Design review of the part built by this model. Coordinates are the model's own, in mm. A direction names the side the tool comes from. Coordinates: 2 decimals unless noted, no trailing zeros. Write each loop counter-clockwise with the first axis right and the second up, starting at its lowest first coordinate (ties: lowest second). Pieces come first, ordered by that corner, then holes. Notation, with made-up numbers: (48, -8) -> (72, -8) arc R17 cw to (72, 17) -> close; hole circle Ø5 at (5, 59.5). An arc over 180 degrees is marked (long way). One line per question, with ' | ' between items. Start each with the question number.
Q1. Add section A-A on x = -1.7. State the section outline as (y, z) points.
Q2. Add section C-C on y = 6.5. State the section outline as (x, z) points.
Q3. Add section B-B on z = 30. State the section outline as (x, y) points, and give its area (3 significant figures).
Q4. Add section D-D on y = 33. State the section outline as (x, z) points.
Q5. For faces 4 (the cylindrical face through (-1.014, 27.683, -34.52)), 5 (the cylindrical face through (-1.014, 37.683, 53.485)), list the 3-axis set-ups (+Z, -Z, +X, -X, +Y, -Y) from which the entire face can be reached by the end or side of a thin tool; tool diameter is ignored.
Q6. Draft analysis for pull direction Y (two halves, no side actions). For faces 1 (the flat face through (-1, 39.325, -1)), 2 (the cylindrical face through (-1.014, -11.689, 9.026)), 3 (the flat face through (-2, 30, 1)), state which applies: pulls with the +Y half, pulls with the -Y half, needs draft (parallel to the pull), parting line crosses it, or undercut.
Q7. Wall thickness on probe 1 along Y at (x, z) = (-0.6, 1.5); probe 2 along Z at (x, y) = (-1.15, 17); probe 3 along Y at (x, z) = (-1.2, 10.5): over which ranges is each line inside the solid? List them lowest first.
from build123d import *

# Parameters (mm, degrees)
BASE_FLANGE1_DEPTH = 2
FILLET1_R          = 3


# Sheet-metal steps are written as plain solids
with BuildPart() as part:
    # Sketch1 → Base-Flange1 (new body)
    with BuildSketch(Plane(origin=(0, 0, 0), x_dir=(0, 0, -1), z_dir=(1, 0, 0))):
        Polygon((-14.5, -22.025862069), (14.5, -22.025862069), (56.5, 39.324712644), (-56.5, 39.324712644), align=None)
        Polygon((-9.227058078, -12.025862069), (9.227058078, -12.025862069), (37.5352548, 29.324712644), (-37.5352548, 29.324712644), align=None, mode=Mode.SUBTRACT)
    extrude(amount=-BASE_FLANGE1_DEPTH)

    # Fillet1
    fillet1_edges = [part.edges().sort_by_distance(p)[0] for p in [
        (-1, 29.324712644, -37.5352548),
        (-1, -12.025862069, -9.227058078),
        (-1, -12.025862069, 9.227058078),
        (-1, 29.324712644, 37.5352548),
        (-1, -22.025862069, -14.5),
        (-1, -22.025862069, 14.5),
        (-1, 39.324712644, 56.5),
        (-1, 39.324712644, -56.5),
    ]]
    fillet(fillet1_edges, radius=FILLET1_R)


solid = part.part
Output values:
1) outline: (-22.03, -12.92) arc R3 ccw to (-20.72, -15.39) -> (34.63, -53.29) arc R3 ccw to (39.32, -50.81) -> (39.32, 50.81) arc R3 ccw to (34.63, 53.29) -> (-20.72, 15.39) arc R3 ccw to (-22.03, 12.92) -> close; hole (-12.03, -7.65) arc R3 ccw to (-10.72, -10.12) -> (24.63, -34.32) arc R3 ccw to (29.32, -31.85) -> (29.32, 31.85) arc R3 ccw to (24.63, 34.32) -> (-10.72, 10.12) arc R3 ccw to (-12.03, 7.65) -> close
2) outline: (-2, -34.03) -> (0, -34.03) -> (0, -21.91) -> (-2, -21.91) -> close; (-2, 21.91) -> (0, 21.91) -> (0, 34.03) -> (-2, 34.03) -> close
3) outline: (-2, 0.62) -> (0, 0.62) -> (0, 18.32) -> (-2, 18.32) -> close; (-2, 29.32) -> (0, 29.32) -> (0, 39.32) -> (-2, 39.32) -> close | area: 55.4 mm2
4) outline: (-2, -52.17) -> (0, -52.17) -> (0, 52.17) -> (-2, 52.17) -> close
5) face 4: +X, -X | face 5: +Z, +X, -X
6) face 1: pulls with the +Y half | face 2: undercut | face 3: needs draft
7) probe 1: y = -22.03 to -12.03, 29.32 to 39.32 | probe 2: z = -41.22 to -29.1, 29.1 to 41.22 | probe 3: y = -22.03 to -10.17, 29.32 to 39.32
